```python
from build123d import *

# Parameters (mm, degrees)
SKETCH1_R               = 17.5
SKETCH1_R_2             = 5
BOSS_EXTRUDE1_DEPTH     = 12
CUT_EXTRUDE1_REACH      = 32.208
SKETCH2_W               = 40
SKETCH2_H               = 15
CUT_EXTRUDE2_REACH      = 32.208
CUT_EXTRUDE2_END_RADIUS = 17.5
SKETCH3_R               = 1.6
SKETCH5_R               = 3.25
CUT_EXTRUDE3_DEPTH      = 7.5
SKETCH8_R               = 1.6
CUT_EXTRUDE4_DEPTH      = 28.50454525


with BuildPart() as part:
    # Sketch1 → Boss-Extrude1 (new body)
    with BuildSketch(Plane(origin=(0, 0, 0), x_dir=(1, 0, 0), z_dir=(0, 1, 0))):
        with Locations(Location((0, 0, 0), (0, 0, 270))):
            Circle(SKETCH1_R)
        with Locations(Location((0, 0, 0), (0, 0, 270))):
            Circle(SKETCH1_R_2, mode=Mode.SUBTRACT)
    extrude(amount=BOSS_EXTRUDE1_DEPTH)

    # Sketch2 → Cut-Extrude1 (cut, up to next)
    with BuildSketch(Plane.XY.offset(-4), mode=Mode.PRIVATE) as cut_extrude1_sk1:
        with Locations((-0.027437806, 7.5)):
            Rectangle(SKETCH2_W, SKETCH2_H)
    cut_extrude1_tool1 = extrude(cut_extrude1_sk1.sketch, amount=-CUT_EXTRUDE1_REACH, mode=Mode.PRIVATE) & part.part
    add(cut_extrude1_tool1.solids().sort_by_distance((-0.027438, 7.5, -4))[0], mode=Mode.SUBTRACT)

    # Cut-Extrude2: up to this cylinder (the profile starts inside it)
    cut_extrude2_end = Plane(origin=(0, 6, 0), z_dir=(0, -1, 0)) * Cylinder(CUT_EXTRUDE2_END_RADIUS, 100.416, mode=Mode.PRIVATE)
    # Sketch3 → Cut-Extrude2 (cut, up to the surface)
    with BuildSketch(Plane(origin=(0, 0, -4), x_dir=(-1, 0, 0), z_dir=(0, 0, -1)), mode=Mode.PRIVATE) as cut_extrude2_sk1:
        with Locations((-12.018362519, 6)):
            Circle(SKETCH3_R)
    cut_extrude2_tool1 = extrude(cut_extrude2_sk1.sketch, amount=-CUT_EXTRUDE2_REACH, mode=Mode.PRIVATE) & cut_extrude2_end
    add(cut_extrude2_tool1.solids().sort_by_distance((12.018363, 6, -4))[0], mode=Mode.SUBTRACT)
    # Sketch3 → Cut-Extrude2 (cut, up to the surface)
    with BuildSketch(Plane(origin=(0, 0, -4), x_dir=(-1, 0, 0), z_dir=(0, 0, -1)), mode=Mode.PRIVATE) as cut_extrude2_sk2:
        with Locations((12.018362519, 6)):
            Circle(SKETCH3_R)
    cut_extrude2_tool2 = extrude(cut_extrude2_sk2.sketch, amount=-CUT_EXTRUDE2_REACH, mode=Mode.PRIVATE) & cut_extrude2_end
    add(cut_extrude2_tool2.solids().sort_by_distance((-12.018363, 6, -4))[0], mode=Mode.SUBTRACT)

    # Sketch5 → Cut-Extrude3 (cut)
    with BuildSketch(Plane.XY.offset(17.5)):
        with Locations((-12.018362519, 6)):
            Circle(SKETCH5_R)
        with Locations((12.018362519, 6)):
            Circle(SKETCH5_R)
    extrude(amount=-CUT_EXTRUDE3_DEPTH, mode=Mode.SUBTRACT)

    # Sketch8 → Cut-Extrude4 (cut, through all)
    with BuildSketch(Plane(origin=(0, 12, 0), x_dir=(1, 0, 0), z_dir=(0, 1, 0))):
        with Locations(Location((-7.5, 0, 0), (0, 0, 270))):
            Circle(SKETCH8_R)
        with Locations(Location((7.5, 0, 0), (0, 0, 270))):
            Circle(SKETCH8_R)
        with Locations(Location((0, -7.5, 0), (0, 0, 270))):
            Circle(SKETCH8_R)
    extrude(amount=-CUT_EXTRUDE4_DEPTH, mode=Mode.SUBTRACT)


solid = part.part
```
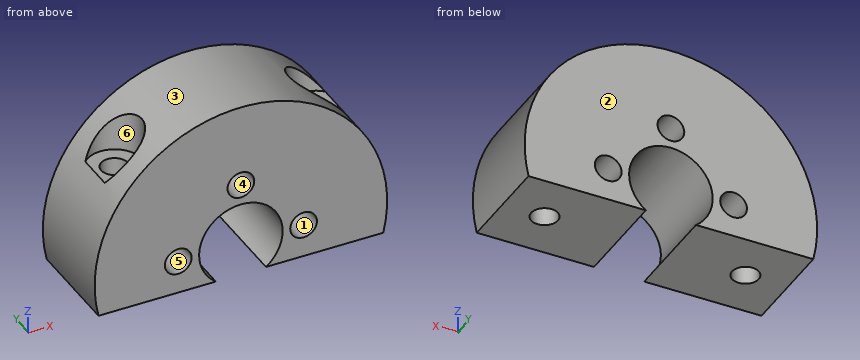
Geometry: final body of the model. Coordinates: model frame, mm. Face numbers are marked on the shaded views. A direction names the side the tool comes from. Coordinates: 2 decimals unless noted, no trailing zeros. Order: outer loops, then holes, each group sorted by start corner. A loop starts at its lowest first (then second) coordinate and runs counter-clockwise, first axis right, second up. Notation, with made-up numbers: (-15, -38) -> (9, -38) arc R14 ccw to (9, -20) -> close; hole circle Ø5 at (-13.5, -37). An arc over 180 degrees is marked (long way). Use CSV: the item, a comma, the result in double quotes.
1) Access query for the marked faces 5 and 6. Directions: +Z, -Z, +X, -X, +Y, -Y. A direction counts if a zero-diameter tool reaches every point of the face in a straight line with its end or side. Return the directions, or none.
Findings:
face 5,"+Y, -Y"
face 6,"+Z"
2) Section A-A on y = 6. Output: boundary loops of the cut face in (x, z), then the cut area to 3 significant figures.
Findings:
outline,"(-17.04, -4) -> (-13.62, -4) -> (-13.62, 10) -> (-14.36, 10) arc R17.5 ccw to start; (-10.42, -4) -> (-3, -4) arc R5 cw (long way) to (3, -4) -> (10.42, -4) -> (10.42, 10) -> (8.77, 10) -> (8.77, 15.14) arc R17.5 ccw to (-8.77, 15.14) -> (-8.77, 10) -> (-10.42, 10) -> close; (13.62, -4) -> (17.04, -4) arc R17.5 ccw to (14.36, 10) -> (13.62, 10) -> close; hole circle Ø3.2 at (-7.5, 0); hole circle Ø3.2 at (0, 7.5); hole circle Ø3.2 at (7.5, 0)"
area,"399 mm^2"
3) Section D-D on z = 12.5. Output: boundary loops of the cut face in (x, y).
Findings:
outline,"(-12.25, 0) -> (12.25, 0) -> (12.25, 2.76) arc R3.25 cw (long way) to (12.25, 9.24) -> (12.25, 12) -> (-12.25, 12) -> (-12.25, 9.24) arc R3.25 cw (long way) to (-12.25, 2.76) -> close"
4) Mould query, pull axis X, two halves, no side actions, for the marked faces 1, 2, 3 and 4. Classes: +X half, -X half, draft (parallel to the pull), parting line (faces both ways), or undercut.
Findings:
face 1,"undercut"
face 2,"draft"
face 3,"parting line"
face 4,"undercut"
5) Pin query (flat end, axial travel): pin 1 Ø1 at (y, z) = (5, 14.5) entering from +X; pin 2 Ø1.7 at (x, y) = (-11.5, 7.5) entering from +Z; pin 3 Ø3 at (x, y) = (-12.02, 6) entering from -Z. Return the tip coordinate at first contact, or that it passes through.
Findings:
pin 1,"stops at x = 9.14"
pin 2,"stops at z = 10"
pin 3,"passes through"
6) Line query: line 1 (X direction, y = 9, z = 0); line 2 (X direction, y = 7, z = 0); line 3 (X direction, y = 6, z = 13.8). Output: solid intervals per line, ascending.
Findings:
line 1,"x = -17.5 to -9.1, -5.9 to -5, 5 to 5.9, 9.1 to 17.5"
line 2,"x = -17.5 to -13.27, -10.77 to -9.1, -5.9 to -5, 5 to 5.9, 9.1 to 10.77, 13.27 to 17.5"
line 3,"x = -8.77 to 8.77"
7) Section B-B on z = 8. Output: boundary loops of the cut face in (x, y).
Findings:
outline,"(-15.56, 0) -> (-1.52, 0) -> (-1.52, 12) -> (-15.56, 12) -> close; (1.52, 0) -> (15.56, 0) -> (15.56, 12) -> (1.52, 12) -> close; hole circle Ø3.2 at (-12.02, 6); hole circle Ø3.2 at (12.02, 6)"
8) Section C-C on x = 0. Output: boundary loops of the cut face in (y, z), then the cut area to 3 significant figures.
Findings:
outline,"(0, 5) -> (12, 5) -> (12, 5.9) -> (0, 5.9) -> close; (0, 9.1) -> (12, 9.1) -> (12, 17.5) -> (0, 17.5) -> close"
area,"112 mm^2"
